Drawing for the job (mm, zero at the part's lowest x, y, z). A direction names the side the tool comes from. Give positions to 0.01 mm unless a question says otherwise; leave off trailing zeros. Write each loop counter-clockwise with the first axis right and the second up, starting at its lowest first coordinate (ties: lowest second). Pieces come first, ordered by that corner, then holes. Notation, with made-up numbers: (-29, 83.25) - (-13, 83.25) arc R26 ccw to (-13, 99.25) - close; hole circle Ø3 at (72.5, 15.25). An arc over 180 degrees is marked (long way). Use CSV: the item, a comma, the result in double quotes.
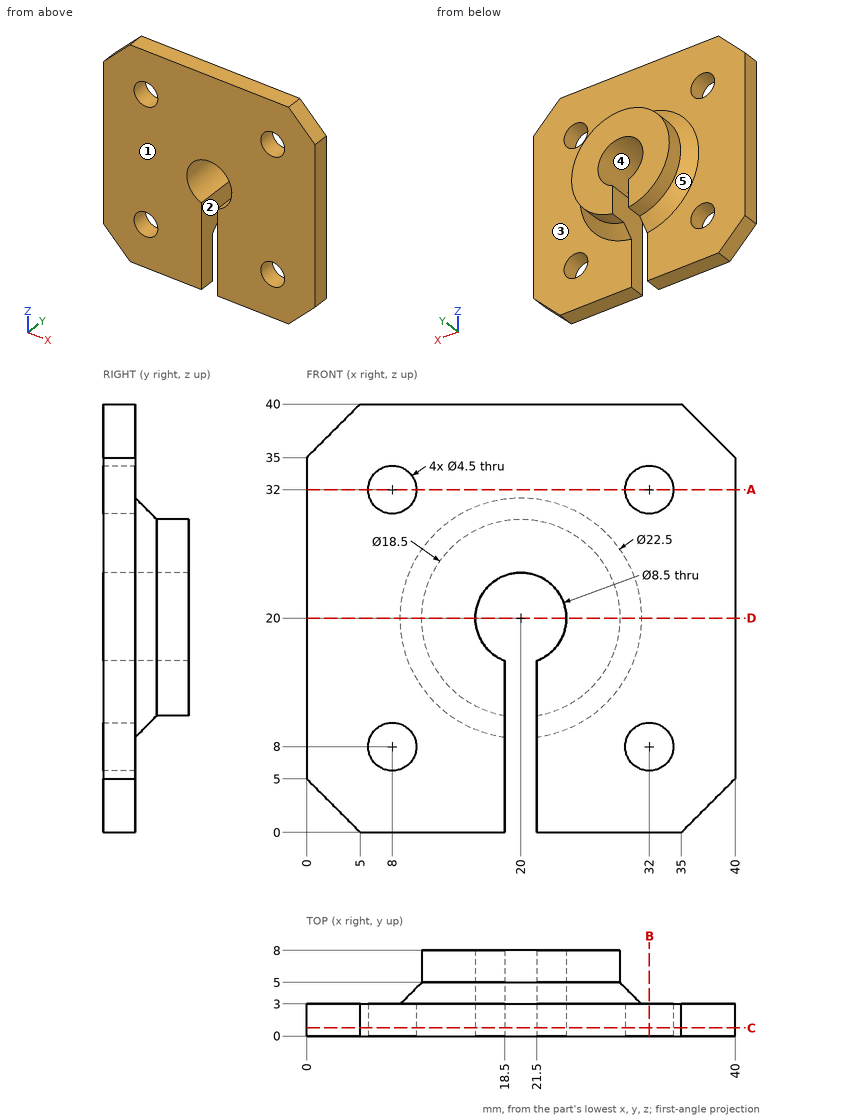
(1) Saw through at B-B, the plane x = 32. List the corners of the cut face in (y, z), then the cut area to 3 significant figures.
Checked values:
outline,"(0, 0) - (3, 0) - (3, 5.75) - (0, 5.75) - close; (0, 10.25) - (3, 10.25) - (3, 29.75) - (0, 29.75) - close; (0, 34.25) - (3, 34.25) - (3, 40) - (0, 40) - close"
area,"93.0 mm^2"
(2) Flat gauge pins, fed straight in: P1, Ø3.5, axis at x = 8, z = 32, coming from the +Y side; P2, Ø6, axis at x = 34, z = 26.5, coming from the +Y side. Where does each tip first touch, or does it go through?
Checked values:
P1,"passes through"
P2,"stops at y = 3"
(3) Saw through at A-A, the plane z = 32. List the corners of the cut face in (x, y).
Checked values:
outline,"(0, 0) - (5.75, 0) - (5.75, 3) - (0, 3) - close; (10.25, 0) - (29.75, 0) - (29.75, 3) - (10.25, 3) - close; (34.25, 0) - (40, 0) - (40, 3) - (34.25, 3) - close"
(4) Saw through at D-D, the plane z = 20. List the corners of the cut face in (x, y), then the cut area to 4 significant figures.
Checked values:
outline,"(0, 0) - (15.75, 0) - (15.75, 8) - (10.75, 8) - (10.75, 5) - (8.75, 3) - (0, 3) - close; (24.25, 0) - (40, 0) - (40, 3) - (31.25, 3) - (29.25, 5) - (29.25, 8) - (24.25, 8) - close"
area,"148.5 mm^2"
(5) Wall check: probe 1 along X at (y, z) = (0.95, 32); probe 2 along X at (y, z) = (2.3, 8); probe 3 along Y at (x, z) = (34.5, 15.5). Give the ranges that are in metal, low to high. Write a range as [from, to].
Checked values:
probe 1,"x = [0, 5.75], [10.25, 29.75], [34.25, 40]"
probe 2,"x = [0, 5.75], [10.25, 18.5], [21.5, 29.75], [34.25, 40]"
probe 3,"y = [0, 3]"
(6) Pull direction X, two halves, no side cores. Call the marked faces 3, 4 and 5: released by +X, released by -X, zero draft, split by the parting line, or undercut.
Checked values:
face 3,"zero draft"
face 4,"undercut"
face 5,"split by the parting line"
(7) Saw through at C-C, the plane y = 0.75. List the corners of the cut face in (x, z).
Checked values:
outline,"(0, 5) - (5, 0) - (18.5, 0) - (18.5, 16.02) arc R4.25 cw (long way) to (21.5, 16.02) - (21.5, 0) - (35, 0) - (40, 5) - (40, 35) - (35, 40) - (5, 40) - (0, 35) - close; hole circle Ø4.5 at (8, 8); hole circle Ø4.5 at (8, 32); hole circle Ø4.5 at (32, 8); hole circle Ø4.5 at (32, 32)"
(8) 3-axis set-ups, long thin cutter, end or side, ignore diameter. For the marked faces 1 and 2: which of +Z, -Z, +X, -X, +Y, -Y reach the whole face in a straight line?
Checked values:
face 1,"+Z, -Z, +X, -X, -Y"
face 2,"-Z, +Y, -Y"
